from build123d import *

# Parameters (mm, degrees)
BOSS_EXTRUDE1_DEPTH = 10
SKETCH2_R           = 2.5
CUT_EXTRUDE2_DEPTH  = 40.940580867


with BuildPart() as part:
    # Sketch1 → Boss-Extrude1 (new body)
    with BuildSketch(Plane.XY):
        with BuildLine():
            Line((-19.5, 0), (-29.5, 0))
            Line((-29.5, 0), (-29.5, 25))
            Line((-29.5, 25), (29.5, 25))
            Line((29.5, 25), (29.5, 0))
            Line((29.5, 0), (19.5, 0))
            ThreePointArc((19.5, 0), (0, 19.5), (-19.5, 0))
        make_face()
    extrude(amount=BOSS_EXTRUDE1_DEPTH)

    # Sketch2 → Cut-Extrude2 (cut, through all)
    with BuildSketch(Plane(origin=(0, 0, 0), x_dir=(1, 0, 0), z_dir=(0, 1, 0))):
        with Locations(Location((-24.5, -5, 0), (0, 0, 270))):
            Circle(SKETCH2_R)
        with Locations(Location((24.5, -5, 0), (0, 0, 270))):
            Circle(SKETCH2_R)
    extrude(amount=CUT_EXTRUDE2_DEPTH, mode=Mode.SUBTRACT)


solid = part.part
Here's how the part is built. I have some questions about the finished solid (model axes, mm). Round coordinates to 2 decimals unless told otherwise and drop trailing zeros. Loops run counter-clockwise (first coordinate to the right, second up) from the corner with the lowest first, then second, coordinate; pieces in that order, holes last. Notation, with made-up numbers: (52, 6) - (103, 6) arc R24 cw to (103, 23) - close; hole circle Ø5 at (42.5, 85.5). An arc over 180 degrees is marked (long way). One line per question, with ' | ' between items. Start each with the question number.
Q1. We'd pull the mould along X, two halves only. Please class faces 1 (the cylindrical face through (-22.39, 12.32, 6.34)), 2 (the flat face through (29.5, 13, 5)), 3 (the flat face through (0, 21, 0)), 4 (the flat face through (-29.5, 12, 5)): +X half, -X half, draft (parallel to the pull), parting line (faces both ways), or undercut.
Q2. I want a section at C-C (z = 5). Write out the boundary of the cut face in (x, y), then the cut area to 3 significant figures.
Q3. I want a section at A-A (x = -24.5). Write out the boundary of the cut face in (y, z), then the cut area to 3 significant figures.
Q4. I want a section at B-B (y = 13). Write out the boundary of the cut face in (x, z), then the cut area to 3 significant figures.
Q5. Please list where these lines run through material, in increasing order: line 1 (X direction, y = 12, z = 5); line 2 (Z direction, x = 24.5, y = 5.75); line 3 (X direction, y = 9.75, z = 5.25). Write a range as [from, to].
Q6. I want a section at D-D (y = 16.75). Write out the boundary of the cut face in (x, z).
Response values:
1) face 1: undercut | face 2: +X half | face 3: draft | face 4: -X half
2) outline: (-29.5, 0) - (-27, 0) - (-27, 25) - (-29.5, 25) - close; (-22, 0) - (-19.5, 0) arc R19.5 cw to (19.5, 0) - (22, 0) - (22, 25) - (-22, 25) - close; (27, 0) - (29.5, 0) - (29.5, 25) - (27, 25) - close | area: 628 mm²
3) outline: (0, 0) - (25, 0) - (25, 2.5) - (0, 2.5) - close; (0, 7.5) - (25, 7.5) - (25, 10) - (0, 10) - close | area: 125 mm²
4) outline: (-29.5, 0) - (-14.53, 0) - (-14.53, 10) - (-29.5, 10) - close; (14.53, 0) - (29.5, 0) - (29.5, 10) - (14.53, 10) - close; hole circle Ø5 at (-24.5, 5); hole circle Ø5 at (24.5, 5) | area: 260 mm²
5) line 1: x = [-29.5, -27], [-22, -15.37], [15.37, 22], [27, 29.5] | line 2: z = [0, 2.5], [7.5, 10] | line 3: x = [-29.5, -26.99], [-22.01, -16.89], [16.89, 22.01], [26.99, 29.5]
6) outline: (-29.5, 0) - (-9.98, 0) - (-9.98, 10) - (-29.5, 10) - close; (9.98, 0) - (29.5, 0) - (29.5, 10) - (9.98, 10) - close; hole circle Ø5 at (-24.5, 5); hole circle Ø5 at (24.5, 5)
